Check sheet for the modelled part. Datum: model origin and axes. Units: mm. Coordinates: 2 decimals unless noted, no trailing zeros. Order: outer loops, then holes, each group sorted by start corner. A loop starts at its lowest first (then second) coordinate and runs counter-clockwise, first axis right, second up. Notation, with made-up numbers: (36, -34) -> (73, -34) arc R17 ccw to (73, -8) -> close; hole circle Ø4 at (19.25, 3). An arc over 180 degrees is marked (long way). Put each result on its own line as item: value. Start each with the question number.
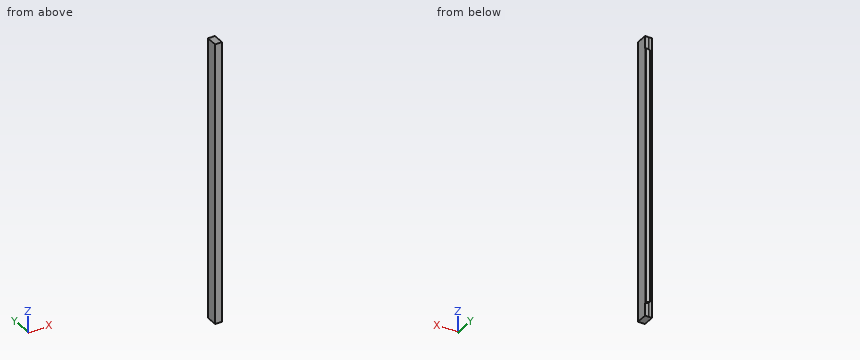
```python
from build123d import *

# Parameters (mm, degrees)
ESQUISSE1_W                  = 30
ESQUISSE1_H                  = 60
BOSS_EXTRU_1_DEPTH           = 1200
ENL_V_MAT_EXTRU_4_DEPTH      = 1202.873537441
ENL_V_MAT_EXTRU_4_DEPTH_BACK = 1202.873537441
ESQUISSE5_W                  = 15
ESQUISSE5_H                  = 10
ENL_V_MAT_EXTRU_2_DEPTH      = 1202.873537441
ENL_V_MAT_EXTRU_2_DEPTH_BACK = 1202.873537441
CONG_1_R                     = 3
ENL_V_MAT_EXTRU_5_REACH      = 1203.416
ESQUISSE7_W                  = 2
ESQUISSE7_H                  = 1200
ENL_V_MAT_EXTRU_6_DEPTH      = 2


with BuildPart() as part:
    # Esquisse1 → Boss.-Extru.1 (new body)
    with BuildSketch(Plane.XY):
        with Locations((15, 30)):
            Rectangle(ESQUISSE1_W, ESQUISSE1_H)
    extrude(amount=BOSS_EXTRU_1_DEPTH)

    # Esquisse5 → Enlèv. mat.-Extru.4 (cut, two sides: drawn at the far end of the back side and taken through both)
    with BuildSketch(Plane.XY.offset(1200).offset(-ENL_V_MAT_EXTRU_4_DEPTH_BACK)):
        with Locations((7.5, 55)):
            Rectangle(ESQUISSE5_W, ESQUISSE5_H)
    extrude(amount=ENL_V_MAT_EXTRU_4_DEPTH + ENL_V_MAT_EXTRU_4_DEPTH_BACK, mode=Mode.SUBTRACT)

    # Esquisse3 → Enlèv. mat.-Extru.2 (cut, two sides: drawn at the far end of the back side and taken through both)
    with BuildSketch(Plane.XY.offset(1200).offset(-ENL_V_MAT_EXTRU_2_DEPTH_BACK)):
        Polygon((15, 60), (30, 54), (30, 60), align=None)
    extrude(amount=ENL_V_MAT_EXTRU_2_DEPTH + ENL_V_MAT_EXTRU_2_DEPTH_BACK, mode=Mode.SUBTRACT)

    # Congé1
    cong_1_edges = [part.edges().sort_by_distance(p)[0] for p in [
        (30, 54, 600),
    ]]
    fillet(cong_1_edges, radius=CONG_1_R)

    # Enlèv. mat.-Extru.5: up to this plane
    enl_v_mat_extru_5_end = Plane(origin=(15, 60, 0), z_dir=(-0.37139067635410367, -0.9284766908852594, 0))
    # Esquisse6 → Enlèv. mat.-Extru.5 (cut, up to the surface)
    with BuildSketch(Plane(origin=(0, 50, 0), x_dir=(1, 0, 0), z_dir=(0, 1, 0)), mode=Mode.PRIVATE) as enl_v_mat_extru_5_sk1:
        Polygon((0, -1200), (30, -1200), (30, -1146), (15, -1140), (0, -1140), align=None)
    enl_v_mat_extru_5_tool1 = split(extrude(enl_v_mat_extru_5_sk1.sketch, amount=ENL_V_MAT_EXTRU_5_REACH, mode=Mode.PRIVATE), bisect_by=enl_v_mat_extru_5_end, keep=Keep.BOTH, mode=Mode.PRIVATE)
    add(enl_v_mat_extru_5_tool1.solids().sort_by_distance((14.74359, 50, 1170.717949))[0], mode=Mode.SUBTRACT)
    # Esquisse6 → Enlèv. mat.-Extru.5 (cut, up to the surface)
    with BuildSketch(Plane(origin=(0, 50, 0), x_dir=(1, 0, 0), z_dir=(0, 1, 0)), mode=Mode.PRIVATE) as enl_v_mat_extru_5_sk2:
        Polygon((0, -60), (0, 0), (30, 0), (30, -54), (15, -60), align=None)
    enl_v_mat_extru_5_tool2 = split(extrude(enl_v_mat_extru_5_sk2.sketch, amount=ENL_V_MAT_EXTRU_5_REACH, mode=Mode.PRIVATE), bisect_by=enl_v_mat_extru_5_end, keep=Keep.BOTH, mode=Mode.PRIVATE)
    add(enl_v_mat_extru_5_tool2.solids().sort_by_distance((14.74359, 50, 29.282051))[0], mode=Mode.SUBTRACT)

    # Esquisse7 → Enlèv. mat.-Extru.6 (cut)
    with BuildSketch(Plane(origin=(0, 50, 0), x_dir=(1, 0, 0), z_dir=(0, 1, 0))):
        with Locations((14, -600)):
            Rectangle(ESQUISSE7_W, ESQUISSE7_H)
    extrude(amount=-ENL_V_MAT_EXTRU_6_DEPTH, mode=Mode.SUBTRACT)


solid = part.part
```
1) Scan lines: line 1 along Y through (x, z) = (8.5, 260); line 2 along X through (y, z) = (51, 117.5); line 3 along Y through (x, z) = (28.5, 847). Record each from-to range of solid material in increasing order. Write a range as [from, to].
2) Gauge pin test, flat ends, axial feed: pin 1 (1.6 mm diameter, centred on x = 14, z = 583, fed in from +Y); pin 2 (4.5 mm diameter, centred on x = 25.5, z = 31, fed in from +Y); pin 3 (1 mm diameter, centred on x = 4.5, z = 781, fed in from -Y); pin 4 (14.5 mm diameter, centred on x = 8, z = 818, fed in from +Y). Record the tip position at first contact, or that the pin passes through.
3) Sectioned sample at A-A (z = 908.5). Record the boundary of the cut face in (x, y).
Entries:
1. line 1: y = [0, 50]
1. line 2: x = [15, 30]
1. line 3: y = [0, 54.57]
2. pin 1: stops at y = 48
2. pin 2: stops at y = 50
2. pin 3: stops at y = 0
2. pin 4: stops at y = 60
3. outline: (0, 0) -> (30, 0) -> (30, 51.97) arc R3 ccw to (28.11, 54.75) -> (15, 60) -> (15, 48) -> (13, 48) -> (13, 50) -> (0, 50) -> close
